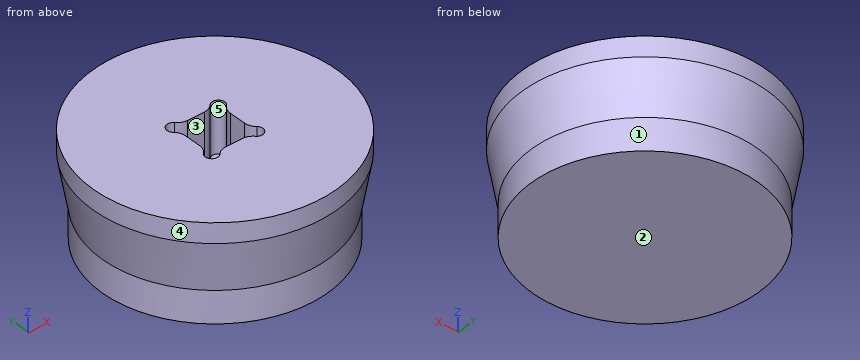
Autodesk Inventor part; units mm, degrees
ref_plane "Plan de construction1" through (0, 0, 4) normal (0, 0, -1) x (-1, 0, 0)
ref_plane "YZ Plane" through (0, 0, 0) normal (1, 0, 0) x (0, 1, 0)
ref_plane "XZ Plane" through (0, 0, 0) normal (0, 1, 0) x (-1, 0, 0)
sketch "Esquisse1" plane through (0, 0, 0) normal (0, 0, 1) x (1, 0, 0)
  circle A0 centre (0, 0) radius 8.85
  dimension "d0" = 17.7
extrude "Extrusion1" add sketch "Esquisse1" along normal blind 7.05 draft 10
sketch "Esquisse2" plane through (0, 0, 7.05) normal (0, 0, 1) x (1, 0, 0)
  line L0 (1.775, -1.775) -> (-1.775, -1.775)
  line L1 (-1.775, -1.775) -> (-1.775, 1.775)
  line L2 (-1.775, 1.775) -> (1.775, 1.775)
  line L3 (1.775, 1.775) -> (1.775, -1.775)
  line L4 (1.775, -1.775) -> (-1.775, 1.775) construction
  line L5 (-1.775, -1.775) -> (1.775, 1.775) construction
  point P0 (0, 0)
  dimension "d3" = 3.55
  dimension "d4" = 3.55
extrude "Extrusion2" cut sketch "Esquisse2" against normal blind 5.5
ref_plane "Plan de construction1" through (0, 0, 4) normal (0, 0, -1) x (-1, 0, 0)
sketch "Esquisse3" plane through (0, 0, 4) normal (0, 0, -1) x (-1, 0, 0)
  circle A0 centre (0, 0) radius 9.5553
  circle A1 centre (0, 0) radius 13.8909
  line L0 (-1.775, 1.775) -> (-1.775, -1.775)
  line L1 (-1.775, -1.775) -> (1.775, -1.775)
  line L2 (1.775, -1.775) -> (1.775, 1.775)
  line L3 (1.775, 1.775) -> (-1.775, 1.775)
extrude "Extrusion3" cut sketch "Esquisse3" against normal through all contours A1
sketch "Esquisse4" plane through (0, 0, 0) normal (0, 0, -1) x (-1, 0, 0)
  circle A0 centre (0, 0) radius 8.85
extrude "Extrusion4" add sketch "Esquisse4" along normal blind 2.5
sketch "Esquisse5" plane through (0, 0, -2.5) normal (0, 0, -1) x (-1, 0, 0)
  line L0 (2.6892, 4.9729) -> (2.6892, -4.9729) construction
  line L1 (2.6892, -4.9729) -> (-2.6892, -4.9729) construction
  line L2 (-2.6892, -4.9729) -> (-2.6892, 4.9729) construction
  line L3 (-2.6892, 4.9729) -> (2.6892, 4.9729) construction
  line L4 (13.3774, 0) -> (-13.3774, 0)
  line L5 (0, -13.3774) -> (0, 13.3774)
  point P0 (0, 0)
  point P1 (-3.9441, 0)
  point P2 (0, -4.9729)
  point P3 (-2.6892, 0)
  point P4 (0, -4.9729)
extrude "Extrusion5" [suppressed]
sketch "Esquisse6" plane through (0, 0, 7.05) normal (0, 0, 1) x (1, 0, 0)
  line L0 (-1.775, 1.775) -> (1.775, 1.775)
  line L1 (1.775, -1.775) -> (-1.775, -1.775)
  point P0 (0, 0)
hole "Perçage1" at (-1.775, 1.775, 7.05) at (1.775, 1.775, 7.05) at (-1.775, -1.775, 7.05) at (1.775, -1.775, 7.05) direction (0, 0, -1) diameter 1 depth 5.5
fillet "Congé1" radius 1 8 edges at (-1.275, 1.775, 4.3) (1.275, 1.775, 4.3) (1.775, 1.275, 4.3) (1.775, -1.275, 4.3) (1.275, -1.775, 4.3) (-1.275, -1.775, 4.3) (-1.775, -1.275, 4.3) (-1.775, 1.275, 4.3)
sketch "Esquisse8" plane through (0, 0, 7.05) normal (0, 0, 1) x (1, 0, 0)
  circle A0 centre (0, 0) radius 10
  dimension "d29" = 20
extrude "Extrusion7" cut sketch "Esquisse8" against normal blind 1.5
sketch "Esquisse7" plane through (0, 0, 7.05) normal (0, 0, 1) x (1, 0, 0)
  arc A0 (3.0373, 1.3601) -> (3.0546, -1.3184) centre (5.8249, 0.0388) ccw construction
  arc A1 (2.6759, 1.5314) -> (2.6954, -1.4944) centre (5.8249, 0.0388) ccw
  arc A2 (3.3988, 1.1887) -> (3.4138, -1.1424) centre (5.8249, 0.0388) ccw
  arc A3 (3.3988, 1.1887) -> (2.6759, 1.5314) centre (3.0373, 1.3601) ccw
  arc A4 (2.6954, -1.4944) -> (3.4138, -1.1424) centre (3.0546, -1.3184) ccw
  point P0 (0, 0)
  dimension "d23" = 0.8
equation "\"d3\" = d4"
properties part number "Power_Button"
Verification items for the finished model (mm, model axes). Face numbers are marked on the shaded views. A direction names the side the tool comes from. Coordinates: 2 decimals unless noted, no trailing zeros. Order: outer loops, then holes, each group sorted by start corner. A loop starts at its lowest first (then second) coordinate and runs counter-clockwise, first axis right, second up.
1. Go/stop test with flat-tipped pins: pin 1 Ø3 at (x, z) = (6.5, 2) entering from -Y; pin 2 Ø4 at (y, z) = (4, -0.5) entering from -X; pin 3 Ø1.1 at (x, z) = (0, 3) entering from -Y. Record where each tip stops, or that it passes through.
Results found:
pin 1: stops at y = -7.78
pin 2: stops at x = -8.65
pin 3: stops at y = -9.48
2. Scan lines: line 1 (X direction, y = 2, z = 2.5); line 2 (Y direction, x = -7.5, z = 1.5); line 3 (Y direction, x = 5, z = 1.25). Record each from-to range of solid material in increasing order.
Results found:
line 1: x = -9.07 to -2.22, -1.29 to 1.29, 2.22 to 9.07
line 2: y = -5.18 to 5.18
line 3: y = -7.57 to 7.57
3. Sectioned sample at C-C, the plane z = 2. Record the cut outline in (x, y) (3 decimals).
Results found:
outline: circle Ø18.405 at (0, 0); hole (-2.108, -1.402) arc R0.5 ccw (long way) to (-1.402, -2.108) arc R1 cw to (-0.657, -1.775) - (0.657, -1.775) arc R1 cw to (1.402, -2.108) arc R0.5 ccw (long way) to (2.108, -1.402) arc R1 cw to (1.775, -0.657) - (1.775, 0.657) arc R1 cw to (2.108, 1.402) arc R0.5 ccw (long way) to (1.402, 2.108) arc R1 cw to (0.657, 1.775) - (-0.657, 1.775) arc R1 cw to (-1.402, 2.108) arc R0.5 ccw (long way) to (-2.108, 1.402) arc R1 cw to (-1.775, 0.657) - (-1.775, -0.657) arc R1 cw to start
4. Sectioned sample at D-D, the plane z = -0.25. Record the cut outline in (x, y).
Results found:
outline: circle Ø17.7 at (0, 0)
5. Sectioned sample at A-A, the plane y = 0. Record the cut outline in (x, z) (3 decimals).
Results found:
outline: (-9.555, 4) - (-8.85, 0) - (-8.85, -2.5) - (8.85, -2.5) - (8.85, 0) - (9.555, 4) - (9.555, 5.55) - (1.775, 5.55) - (1.775, 1.55) - (-1.775, 1.55) - (-1.775, 5.55) - (-9.555, 5.55) - close
6. Set-up check for the marked faces 4 and 5: record each of +Z, -Z, +X, -X, +Y, -Y from which the full face is reachable in a straight line by a thin tool's end or side.
Results found:
face 4: +Z, -Z
face 5: +Z
7. Release check for a two-part mould opening along X. For the marked faces 1, 2 and 3 record: +X half, -X half, draft (parallel to the pull), parting line (faces both ways), or undercut.
Results found:
face 1: parting line
face 2: draft
face 3: undercut
